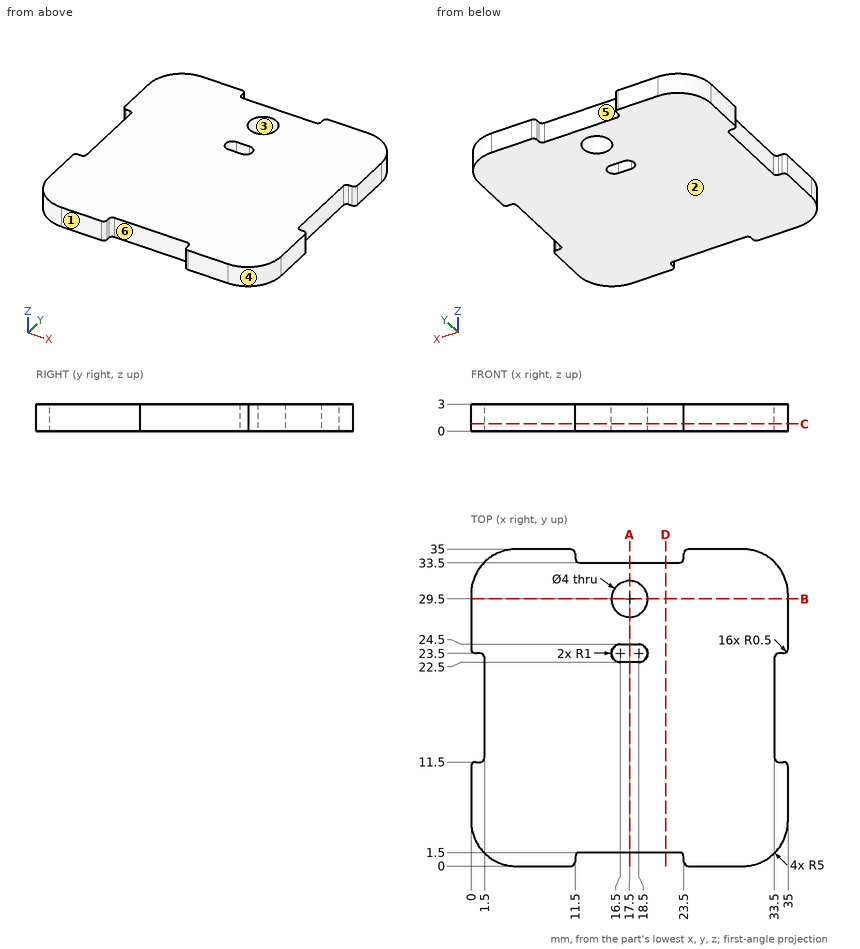
Part print with two shaded views. Sizes in mm from the minimum x, y, z corner. A direction names the side the tool comes from. Round coordinates to 2 decimals unless told otherwise and drop trailing zeros. Order: outer loops, then holes, each group sorted by start corner. A loop starts at its lowest first (then second) coordinate and runs counter-clockwise, first axis right, second up. Notation, with made-up numbers: (1, -39.5) -> (43, -39.5) arc R26 ccw to (43, -1.5) -> close; hole circle Ø7 at (-26, -29). An arc over 180 degrees is marked (long way). Use one line per item in the form item = value.
Item 1: Tool access for the marked faces 4, 5 and 6: list every direction of +Z, -Z, +X, -X, +Y, -Y with a clear straight run to the whole face (end or side of a thin tool).
Returned:
face_4 = +Z, -Z, +X, -Y
face_5 = +Z, -Z, +Y
face_6 = +Z, -Z, -Y
Item 2: Flat gauge pins, fed straight in: pin 1 Ø0.9 at (y, z) = (17, 2) entering from -X; pin 2 Ø0.6 at (y, z) = (0.5, 2) entering from +X; pin 3 Ø0.6 at (y, z) = (0.5, 1) entering from -X; pin 4 Ø1.5 at (x, y) = (10.5, 27) entering from -Z. Where does each tip first touch, or does it go through?
Returned:
pin_1 = 1.5
pin_2 = 32.71
pin_3 = 2.29
pin_4 = 0
Item 3: Cut at B-B, the plane y = 29.5. Write the cut outline in (x, z), and give its area (3 significant figures).
Returned:
outline = (0, 0) -> (15.5, 0) -> (15.5, 3) -> (0, 3) -> close; (19.5, 0) -> (35, 0) -> (35, 3) -> (19.5, 3) -> close
area = 93.0 mm^2
Item 4: Drill centre lines: line 1 (Y direction, x = 17.5, z = 0.75); line 2 (Y direction, x = 16.5, z = 1.5); line 3 (Y direction, x = 13, z = 0.6). Where is each one in solid material? Low to high.
Returned:
line_1 = 1.5 to 22.5, 24.5 to 27.5, 31.5 to 33.5
line_2 = 1.5 to 22.5, 24.5 to 27.77, 31.23 to 33.5
line_3 = 1.5 to 33.5
Item 5: Cut at D-D, the plane x = 21.5. Write the cut outline in (y, z), and give its area (3 significant figures).
Returned:
outline = (1.5, 0) -> (33.5, 0) -> (33.5, 3) -> (1.5, 3) -> close
area = 96.0 mm^2
Item 6: Cut at A-A, the plane x = 17.5. Write the cut outline in (y, z).
Returned:
outline = (1.5, 0) -> (22.5, 0) -> (22.5, 3) -> (1.5, 3) -> close; (24.5, 0) -> (27.5, 0) -> (27.5, 3) -> (24.5, 3) -> close; (31.5, 0) -> (33.5, 0) -> (33.5, 3) -> (31.5, 3) -> close
Item 7: Cut at C-C, the plane z = 0.8. Give the number of separate pieces and of enclosed holes in the cut face, and give its area (3 significant figures).
Returned:
separate_pieces = 1
enclosed_holes = 2
area = 1,110 mm^2
Item 8: Pull direction Y, two halves, no side cores. Call the marked faces 1, 2 and 3: released by +Y, released by -Y, zero draft, split by the parting line, or undercut.
Returned:
face_1 = released by -Y
face_2 = zero draft
face_3 = undercut
